from build123d import *

# Parameters (mm, degrees)
BOSS_EXTRUDE1_DEPTH = 50


with BuildPart() as part:
    # Sketch1 → Boss-Extrude1 (new, symmetric)
    with BuildSketch(Plane(origin=(0, 0, 0), x_dir=(0, 0, -1), z_dir=(1, 0, 0))):
        with BuildLine():
            Line((-4, 3.746468452), (-4, -46.253531548))
            ThreePointArc((-4, -46.253531548), (-2.623401872, -49.57693342), (0.7, -50.953531548))
            Line((0.7, -50.953531548), (20.7, -50.953531548))
            Line((20.7, -50.953531548), (20.7, -48.953531548))
            Line((20.7, -48.953531548), (0.7, -48.953531548))
            ThreePointArc((0.7, -48.953531548), (-1.209188309, -48.162719858), (-2, -46.253531548))
            Line((-2, -46.253531548), (-2, 3.746468452))
            Line((-2, 3.746468452), (-4, 3.746468452))
        make_face()
    extrude(amount=BOSS_EXTRUDE1_DEPTH, both=True)


solid = part.part
Verification items for the finished model (mm, model axes). A direction names the side the tool comes from. Coordinates: 2 decimals unless noted, no trailing zeros. Write each loop counter-clockwise with the first axis right and the second up, starting at its lowest first coordinate (ties: lowest second). Pieces come first, ordered by that corner, then holes. Notation, with made-up numbers: M 34.25,64.5 L 62.25,64.5 A9 ccw 62.25,80.5 Z; hole C -32.5,-34 d4. An arc over 180 degrees is marked long. Use a Markdown table: item, result.
Q1. Set-up check for faces 4 (the face through (1, -48.954, -11)), 5 (the face through (1, 3.746, 3)): record each of +Z, -Z, +X, -X, +Y, -Y from which the full face is reachable in a straight line by a thin tool's end or side.
Reply:
| item | result |
|---|---|
| face 4 | -Z, +X, -X, +Y |
| face 5 | +Z, -Z, +X, -X, +Y |
Q2. Thickness scan on line 1 (Z direction, x = -40, y = -31); line 2 (Y direction, x = -44.5, z = -14.25); line 3 (Z direction, x = 38, y = -47.5). Record the ranges inside material, lowest first.
Reply:
| item | result |
|---|---|
| line 1 | z = 2 to 4 |
| line 2 | y = -50.95 to -48.95 |
| line 3 | z = 1.7 to 3.83 |
Q3. Go/stop test with flat-tipped pins: P1, Ø8, axis at y = -42.5, z = -8, coming from the +X side; P2, Ø25, axis at x = 19.5, y = -30, coming from the -Z side; P3, Ø1.5, axis at x = -11, z = -9.5, coming from the +Y side. Record where each tip stops, or that it passes through.
Reply:
| item | result |
|---|---|
| P1 | passes through |
| P2 | stops at z = 2 |
| P3 | stops at y = -48.95 |
Q4. Sectioned sample at A-A, the plane x = 44.5. Record the boundary of the cut face in (y, z).
Reply:
| item | result |
|---|---|
| outline | M -50.95,-20.7 L -48.95,-20.7 L -48.95,-0.7 A2.7 cw -46.25,2 L 3.75,2 L 3.75,4 L -46.25,4 A4.7 ccw -50.95,-0.7 Z |
Q5. Sectioned sample at C-C, the plane y = -28.5. Record the boundary of the cut face in (x, z), plus the area to 3 significant figures.
Reply:
| item | result |
|---|---|
| outline | M -50,2 L 50,2 L 50,4 L -50,4 Z |
| area | 200 mm² |
Q6. Sectioned sample at B-B, the plane z = -7.75. Record the boundary of the cut face in (x, y), plus the area to 3 significant figures.
Reply:
| item | result |
|---|---|
| outline | M -50,-50.95 L 50,-50.95 L 50,-48.95 L -50,-48.95 Z |
| area | 200 mm² |
Q7. Draft check along X on faces 1 (the face through (1, -50, -20.7)), 2 (the face through (50, -32, 3)), 3 (the face through (-50, -32, 3)). Enter one of: +X half, -X half, draft (parallel to the pull), parting line (faces both ways), or undercut.
Reply:
| item | result |
|---|---|
| face 1 | draft |
| face 2 | +X half |
| face 3 | -X half |
